Autodesk Inventor part; units mm, degrees
ref_plane "YZ Plane" through (0, 0, 0) normal (1, 0, 0) x (0, 1, 0)
ref_plane "XZ Plane" through (0, 0, 0) normal (0, 1, 0) x (-1, 0, 0)
ref_plane "XY Plane" through (0, 0, 0) normal (0, 0, 1) x (1, 0, 0)
sketch "スケッチ1" plane through (0, 0, 0) normal (0, 0, 1) x (1, 0, 0)
  line L0 (-35, -50) -> (35, -50)
  line L1 (35, -50) -> (35, 50)
  line L2 (35, 50) -> (-35, 50)
  line L3 (-35, 50) -> (-35, -50)
  line L4 (-35, -50) -> (35, 50) construction
  line L5 (35, -50) -> (-35, 50) construction
  point P0 (0, 0)
  dimension "d0" = 70
  dimension "d1" = 100
extrude "押し出し1" add sketch "スケッチ1" along normal blind 3
sketch "スケッチ2" plane through (0, 0, 3) normal (0, 0, 1) x (1, 0, 0)
  line L0 (-35, -50) -> (35, -50)
  point P0 (0, 0)
  point P1 (0, -40)
  point P2 (0, -10)
  dimension "d4" = 10
  dimension "d5" = 30
hole "穴1" at (0, -40, 3) at (0, -10, 3) direction (0, 0, -1) diameter 3.2 depth 8.8 tip angle 118
sketch "スケッチ3" plane through (0, 0, 3) normal (0, 0, 1) x (1, 0, 0)
  line L0 (-35, 50) -> (-35, -50)
  line L1 (35, -50) -> (35, 50)
  point P0 (0, 0)
  point P1 (-28, 25.3325)
  point P2 (28, 25.3325)
  point P3 (-28, -4.6675)
  point P4 (28, -4.6675)
  dimension "d14" = 7
  dimension "d15" = 7
  dimension "d16" = 30
  dimension "d17" = 30
  dimension "d18" = 56
hole "穴2" at (-28, 25.3325, 3) at (28, 25.3325, 3) at (-28, -4.6675, 3) at (28, -4.6675, 3) direction (0, 0, -1) diameter 2.459 depth 8.8 tip angle 118
properties part number "20220613_カメラ固定"
Check sheet for the modelled part. Datum: model origin and axes. Units: mm. Round coordinates to 2 decimals unless told otherwise and drop trailing zeros. Loops run counter-clockwise (first coordinate to the right, second up) from the corner with the lowest first, then second, coordinate; pieces in that order, holes last. Notation, with made-up numbers: (-1.5, 55) - (24.5, 55) arc R29 ccw to (24.5, 94) - close; hole circle Ø6 at (64.25, 17). An arc over 180 degrees is marked (long way). Answer as CSV lines item,"result". Start each with the question number.
Item 1: Scan lines: line 1 (Y direction, x = 0, z = 1.15); line 2 (Y direction, x = 28, z = 0.7); line 3 (X direction, y = -4.5, z = 2.4). Record each from-to range of solid material in increasing order. Write a range as [from, to].
Item 2: Section check B-B (x = -28). Record the boundary of the cut face in (y, z).
Item 3: Section check A-A (x = 0). Record the boundary of the cut face in (y, z), and give its area (3 significant figures).
Item 4: Release check for a two-part mould opening along Y. For faces 1 (the cylindrical face through (-1.08, -38.82, 1.48)), 2 (the flat face through (0, 1, 3)), 3 (the flat face through (0, -50, 1)) record: +Y half, -Y half, draft (parallel to the pull), parting line (faces both ways), or undercut.
Report:
1,line 1,"y = [-50, -41.6], [-38.4, -11.6], [-8.4, 50]"
1,line 2,"y = [-50, -5.9], [-3.44, 24.1], [26.56, 50]"
1,line 3,"x = [-35, -29.22], [-26.78, 26.78], [29.22, 35]"
2,outline,"(-50, 0) - (-5.9, 0) - (-5.9, 3) - (-50, 3) - close; (-3.44, 0) - (24.1, 0) - (24.1, 3) - (-3.44, 3) - close; (26.56, 0) - (50, 0) - (50, 3) - (26.56, 3) - close"
3,outline,"(-50, 0) - (-41.6, 0) - (-41.6, 3) - (-50, 3) - close; (-38.4, 0) - (-11.6, 0) - (-11.6, 3) - (-38.4, 3) - close; (-8.4, 0) - (50, 0) - (50, 3) - (-8.4, 3) - close"
3,area,"281 mm2"
4,face 1,"undercut"
4,face 2,"draft"
4,face 3,"-Y half"
